from build123d import *

# Parameters (mm, degrees)
SKETCH_R      = 15
PAD_DEPTH     = 4
SKETCH001_R   = 1.5
PAD001_DEPTH  = 2
SKETCH002_R   = 15
SKETCH002_R_2 = 14
PAD002_DEPTH  = 5
SKETCH003_W   = 50
SKETCH003_H   = 50
PAD003_DEPTH  = 2
SKETCH004_W   = 50
SKETCH004_H   = 50
SKETCH004_W_2 = 46
SKETCH004_H_2 = 46
PAD004_DEPTH  = 10


with BuildPart() as part:
    # Sketch → Pad (new body)
    with BuildSketch(Plane.XY):
        Circle(SKETCH_R)
    extrude(amount=PAD_DEPTH)

    # Sketch001 → Pad001 (join)
    with BuildSketch(Plane.XY):
        with BuildLine():
            add(Edge.make_bspline(
                [(-6.970964, 13.281779), (-4.960107, 17.400153), (0, 20.361549), (4.960107, 17.400153), (6.970964, 13.281779)],
                knots=[0, 0, 0, 0, 0.5, 1, 1, 1, 1], degree=3))
            Line((6.970964, 13.281779), (-6.970964, 13.281779))
        make_face()
        with Locations((0, 16.734485)):
            Circle(SKETCH001_R, mode=Mode.SUBTRACT)
    extrude(amount=PAD001_DEPTH)

    # Sketch002 → Pad002 (join)
    with BuildSketch(Plane.XY):
        Circle(SKETCH002_R)
        Circle(SKETCH002_R_2, mode=Mode.SUBTRACT)
    extrude(amount=PAD002_DEPTH)

    # Sketch003 → Pad003 (join)
    with BuildSketch(Plane.XY):
        Rectangle(SKETCH003_W, SKETCH003_H)
    extrude(amount=-PAD003_DEPTH)

    # Sketch004 → Pad004 (join)
    with BuildSketch(Plane.XY):
        Rectangle(SKETCH004_W, SKETCH004_H)
        Rectangle(SKETCH004_W_2, SKETCH004_H_2, mode=Mode.SUBTRACT)
    extrude(amount=PAD004_DEPTH)


solid = part.part
The model under review builds one solid part; all positions refer to its coordinate system, in mm. A direction names the side the tool comes from. Round coordinates to 2 decimals unless told otherwise and drop trailing zeros. Order: outer loops, then holes, each group sorted by start corner. A loop starts at its lowest first (then second) coordinate and runs counter-clockwise, first axis right, second up. Notation, with made-up numbers: (24, 63.25) -> (55, 63.25) arc R12 ccw to (55, 75.25) -> close; hole circle Ø2 at (53.25, 53). An arc over 180 degrees is marked (long way). Return JSON: item names as keys, results as strings.
1. The part is to be moulded in two halves that separate along X. For faces 1 (the face through (0, -23, 5)), 2 (the face through (0, 25, 4)), 3 (the face through (-25, 0, 4)), say which applies: +X half, -X half, draft (parallel to the pull), parting line (faces both ways), or undercut.
Answer block:
{"face 1": "undercut", "face 2": "draft", "face 3": "-X half"}
2. Take a section at C-C (y = 0). Write out the cut boundary in (x, z).
Answer block:
{"outline": "(-25, -2) -> (25, -2) -> (25, 10) -> (23, 10) -> (23, 0) -> (15, 0) -> (15, 5) -> (14, 5) -> (14, 4) -> (-14, 4) -> (-14, 5) -> (-15, 5) -> (-15, 0) -> (-23, 0) -> (-23, 10) -> (-25, 10) -> close"}
3. For L1, parallel to Y at x = 0, z = 1.05; L2, parallel to X at y = 0, z = 4.55; L3, parallel to X at y = 0.5, z = 9.75, list the stretches that pass through material, from the lowest coordinate up. Write a range as [from, to].
Answer block:
{"L1": "y = [-25, -23], [-15, 15.23], [18.23, 18.88], [23, 25]", "L2": "x = [-25, -23], [-15, -14], [14, 15], [23, 25]", "L3": "x = [-25, -23], [23, 25]"}
4. Take a section at A-A (z = 9). Write out the cut boundary in (x, y).
Answer block:
{"outline": "(-25, -25) -> (25, -25) -> (25, 25) -> (-25, 25) -> close; hole (-23, -23) -> (23, -23) -> (23, 23) -> (-23, 23) -> close"}
5. Take a section at B-B (x = 19.5). Write out the cut boundary in (y, z).
Answer block:
{"outline": "(-25, -2) -> (25, -2) -> (25, 10) -> (23, 10) -> (23, 0) -> (-23, 0) -> (-23, 10) -> (-25, 10) -> close"}
6. Insertion check: P1, Ø4, axis at x = -13, y = -8, coming from the +Z side; P2, Ø5, axis at x = -6, y = -19.5, coming from the +Z side; P3, Ø1.7, axis at x = 2.5, y = 16.5, coming from the +Z side. Each pin has a flat end and moves straight along its axis. Give the tip position at first contact, or say it passes through.
Answer block:
{"P1": "stops at z = 5", "P2": "stops at z = 0", "P3": "stops at z = 2"}
7. For faces 4 (the face through (0, -25, 4)), 5 (the face through (1.1, 15.3, 2)), list the 3-axis set-ups (+Z, -Z, +X, -X, +Y, -Y) from which the entire face can be reached by the end or side of a thin tool; tool diameter is ignored.
Answer block:
{"face 4": "+Z, -Z, +X, -X, -Y", "face 5": "+Z"}
